Geometry check sheet. Reference: the model listing, model coordinates, mm. A direction names the side the tool comes from. Coordinates: 2 decimals unless noted, no trailing zeros. Write each loop counter-clockwise with the first axis right and the second up, starting at its lowest first coordinate (ties: lowest second). Pieces come first, ordered by that corner, then holes. Notation, with made-up numbers: M 64,50.5 L 84,50.5 A34 cw 84,81.5 Z; hole C 1,39 d7. An arc over 180 degrees is marked long. Write each question's results on one line, items separated by ' | '.
```python
from build123d import *

# Parameters (mm, degrees)
F0_W     = 88.9
F0_H     = 165.1
F1_DEPTH = 6.35
F2_DEPTH = 25.4
F3_DEPTH = 50.8
F4_SIZE2 = 12.7
F4_SIZE  = 7.3323484187
F5_SIZE  = 5.08


with BuildPart() as f1:
    # F0 (on Top) → F1 (new body)
    with BuildSketch(Plane.XY):
        with Locations((3.3165217161, -5.8097798109)):
            Rectangle(F0_W, F0_H)
        Polygon((-34.7834782839, 32.2902201891), (-34.7834782839, 70.3902201891), (3.3165217161, 70.3902201891), (41.4165217161, 70.3902201891), (41.4165217161, -43.9097798109), (41.4165217161, -82.0097798109), (3.3165217161, -82.0097798109), (-34.7834782839, -82.0097798109), align=None, mode=Mode.SUBTRACT)
    extrude(amount=F1_DEPTH)

    # F0 (on Top) → F2 (join)
    with BuildSketch(Plane.XY):
        with BuildLine():
            Line((41.4165217161, 70.3902201891), (3.3165217161, 70.3902201891))
            Line((3.3165217161, 70.3902201891), (3.3165217161, 44.9902201891))
            ThreePointArc((3.3165217161, 44.9902201891), (-0.4032221628, 36.009964068), (-9.3834782839, 32.2902201891))
            Line((-9.3834782839, 32.2902201891), (-34.7834782839, 32.2902201891))
            Line((-34.7834782839, 32.2902201891), (-34.7834782839, -82.0097798109))
            Line((-34.7834782839, -82.0097798109), (3.3165217161, -82.0097798109))
            Line((3.3165217161, -82.0097798109), (3.3165217161, -56.6097798109))
            ThreePointArc((3.3165217161, -56.6097798109), (7.036265595, -47.6295236898), (16.0165217161, -43.9097798109))
            Line((16.0165217161, -43.9097798109), (41.4165217161, -43.9097798109))
            Line((41.4165217161, -43.9097798109), (41.4165217161, 70.3902201891))
        make_face()
    extrude(amount=F2_DEPTH)

    # F0 (on Top) → F3 (join)
    with BuildSketch(Plane.XY):
        with BuildLine():
            Line((3.3165217161, 70.3902201891), (-34.7834782839, 70.3902201891))
            Line((-34.7834782839, 70.3902201891), (-34.7834782839, 32.2902201891))
            Line((-34.7834782839, 32.2902201891), (-9.3834782839, 32.2902201891))
            ThreePointArc((-9.3834782839, 32.2902201891), (-0.4032221628, 36.009964068), (3.3165217161, 44.9902201891))
            Line((3.3165217161, 44.9902201891), (3.3165217161, 70.3902201891))
        make_face()
        with BuildLine():
            Line((41.4165217161, -82.0097798109), (41.4165217161, -43.9097798109))
            Line((41.4165217161, -43.9097798109), (16.0165217161, -43.9097798109))
            ThreePointArc((16.0165217161, -43.9097798109), (7.036265595, -47.6295236898), (3.3165217161, -56.6097798109))
            Line((3.3165217161, -56.6097798109), (3.3165217161, -82.0097798109))
            Line((3.3165217161, -82.0097798109), (41.4165217161, -82.0097798109))
        make_face()
    extrude(amount=F3_DEPTH)

    # F4
    f4_edges = [f1.edges().sort_by_distance(p)[0] for p in [
        (22.366522, -82.00978, 50.8),
        (41.416522, -62.95978, 50.8),
    ]]
    f4_side = f1.faces().sort_by_distance((22.762564, -63.355822, 50.8))[0]
    chamfer(f4_edges, length=F4_SIZE, length2=F4_SIZE2, reference=f4_side)

    # F5
    f5_edges = [f1.edges().sort_by_distance(p)[0] for p in [
        (-15.733478, 70.39022, 50.8),
        (-34.783478, 51.34022, 50.8),
    ]]
    chamfer(f5_edges, length=F5_SIZE)


solid = f1.part
```
Q1. Depth check by flat-ended pin: P1, Ø12, axis at x = 5, y = -64, coming from the -Z side; P2, Ø3, axis at x = 9, z = 13, coming from the -Y side; P3, Ø2, axis at y = -36, z = 19, coming from the +X side; P4, Ø8, axis at x = 28.5, z = 23.5, coming from the +Y side. Enter the tip coordinate at first touch or a pass-through.
Geometry check:
P1: stops at z = 0 | P2: stops at y = -82.01 | P3: stops at x = 41.42 | P4: stops at y = 70.39
Q2. Access from +Z, -Z, +X, -X, +Y, -Y to the whole of each face (thin tool, end or side, straight path). Record for faces 1 (the flat face through (3.317, 58, 38)), 2 (the flat face through (41.417, -24, 18)), 3 (the flat face through (3.317, -69, 38)).
Geometry check:
face 1: +Z, +X, +Y | face 2: +Z, +X, +Y, -Y | face 3: +Z, -X, -Y
Q3. Sectioned sample at A-A on z = 28. Record the cut outline in (x, y), and give its area (3 significant figures).
Geometry check:
outline: M -34.78,32.29 L -9.38,32.29 A12.7 ccw 3.32,44.99 L 3.32,70.39 L -34.78,70.39 Z; M 3.32,-82.01 L 41.42,-82.01 L 41.42,-43.91 L 16.02,-43.91 A12.7 ccw 3.32,-56.61 Z | area: 2,830 mm2
Q4. Sectioned sample at C-C on x = -1.5. Record the cut outline in (y, z), and give its area (3 significant figures).
Geometry check:
outline: M -88.36,0 L 76.74,0 L 76.74,6.35 L 70.39,6.35 L 70.39,45.72 L 65.31,50.8 L 35.03,50.8 L 35.03,25.4 L -82.01,25.4 L -82.01,6.35 L -88.36,6.35 Z | area: 4,840 mm2
Q5. Sectioned sample at B-B on y = -47. Record the cut outline in (x, z), and give its area (3 significant figures).
Geometry check:
outline: M -41.13,0 L 47.77,0 L 47.77,6.35 L 41.42,6.35 L 41.42,38.1 L 34.08,50.8 L 7.71,50.8 L 7.71,25.4 L -34.78,25.4 L -34.78,6.35 L -41.13,6.35 Z | area: 2,830 mm2
Q6. Sectioned sample at D-D on z = 14. Record the cut outline in (x, y).
Geometry check:
outline: M -34.78,-82.01 L 41.42,-82.01 L 41.42,70.39 L -34.78,70.39 Z
Q7. Scan lines: probe 1 along X at (y, z) = (59, 40); probe 2 along Y at (x, z) = (22, 13); probe 3 along Z at (x, y) = (-31, -33). Record each from-to range of solid material in increasing order.
Geometry check:
probe 1: x = -34.78 to 3.32 | probe 2: y = -82.01 to 70.39 | probe 3: z = 0 to 25.4
